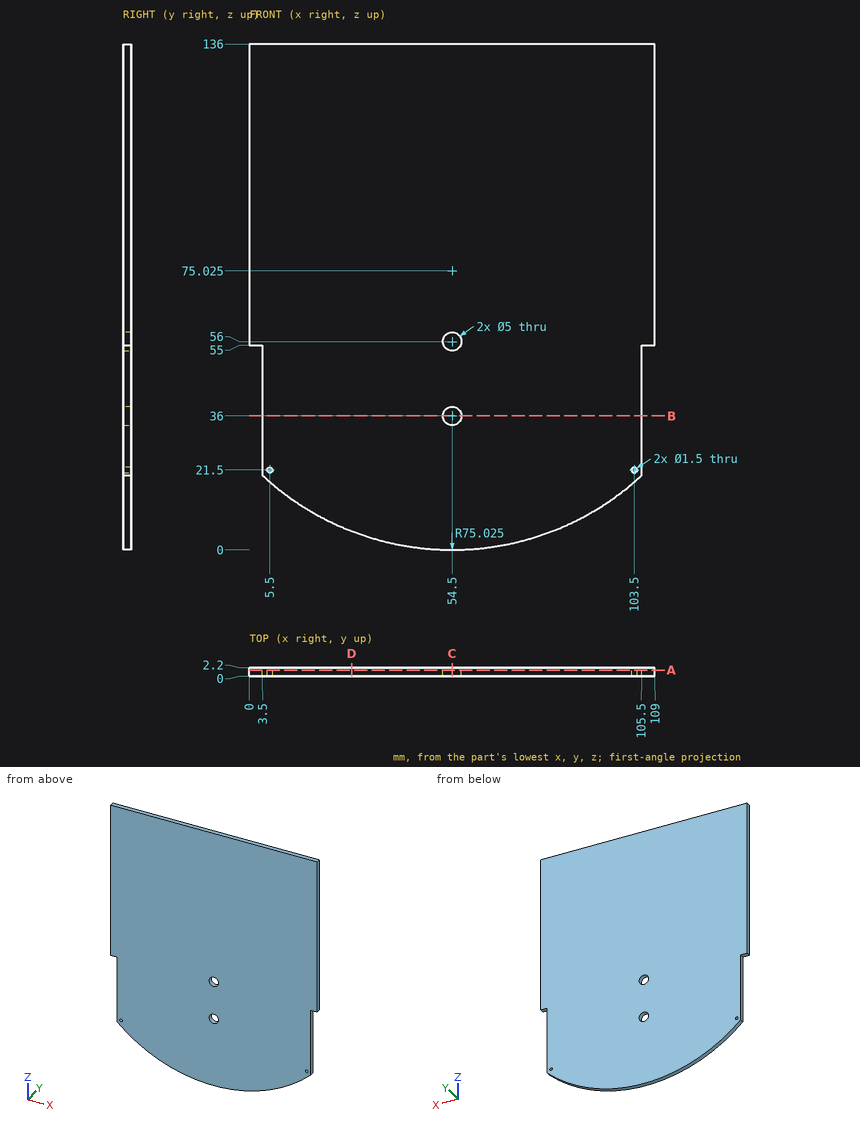
Could you check a few things on this drawing? It's one solid part, dimensions in mm from its lowest x, y, z. Round coordinates to 2 decimals unless told otherwise and drop trailing zeros. Write each loop counter-clockwise with the first axis right and the second up, starting at its lowest first coordinate (ties: lowest second). Pieces come first, ordered by that corner, then holes. Notation, with made-up numbers: (-3, -15) -> (38, -15) arc R12 cw to (38, 7) -> close; hole circle Ø5 at (75.5, 64). An arc over 180 degrees is marked (long way). Use a Markdown table: item, result.
1. If we section it at B-B (z = 36): List the corners of the cut face in (x, y) for me.
Answer key:
| item | result |
|---|---|
| outline | (3.5, 0) -> (52, 0) -> (52, 2.2) -> (3.5, 2.2) -> close; (57, 0) -> (105.5, 0) -> (105.5, 2.2) -> (57, 2.2) -> close |
2. For pin 1 Ø1.1 at (x, y) = (2, 1) entering from -Z; pin 2 Ø3 at (x, z) = (54.5, 56) entering from -Y; pin 3 Ø1.1 at (y, z) = (1, 29.5) entering from -X; pin 4 Ø0.7 at (y, z) = (1.5, 35) entering from +X, each with a flat end and sliding along its axis, tell me the tip position at first contact or that it passes through.
Answer key:
| item | result |
|---|---|
| pin 1 | stops at z = 55 |
| pin 2 | passes through |
| pin 3 | stops at x = 3.5 |
| pin 4 | stops at x = 105.5 |
3. If we section it at A-A (y = 1.55): List the corners of the cut face in (x, z) for me (3 decimals), then the cut area to 3 significant figures.
Answer key:
| item | result |
|---|---|
| outline | (0, 55) -> (3.5, 55) -> (3.5, 20) arc R75.025 ccw to (105.5, 20) -> (105.5, 55) -> (109, 55) -> (109, 136) -> (0, 136) -> close; hole circle Ø1.5 at (5.5, 21.5); hole circle Ø5 at (54.5, 36); hole circle Ø5 at (54.5, 56); hole circle Ø1.5 at (103.5, 21.5) |
| area | 13,800 mm^2 |
4. If we section it at D-D (x = 27.5): List the corners of the cut face in (y, z) for me.
Answer key:
| item | result |
|---|---|
| outline | (0, 5.03) -> (2.2, 5.03) -> (2.2, 136) -> (0, 136) -> close |
5. If we section it at C-C (x = 54.5): List the corners of the cut face in (y, z) for me.
Answer key:
| item | result |
|---|---|
| outline | (0, 0) -> (2.2, 0) -> (2.2, 33.5) -> (0, 33.5) -> close; (0, 38.5) -> (2.2, 38.5) -> (2.2, 53.5) -> (0, 53.5) -> close; (0, 58.5) -> (2.2, 58.5) -> (2.2, 136) -> (0, 136) -> close |
6. Please list where these lines run through material, in increasing order: probe 1 along X at (y, z) = (0.5, 36); probe 2 along X at (y, z) = (1.6, 56); probe 3 along X at (y, z) = (1.8, 22).
Answer key:
| item | result |
|---|---|
| probe 1 | x = 3.5 to 52, 57 to 105.5 |
| probe 2 | x = 0 to 52, 57 to 109 |
| probe 3 | x = 3.5 to 4.94, 6.06 to 102.94, 104.06 to 105.5 |
